```python
from build123d import *

# Parameters (mm, degrees)
SKETCH2_R               = 19.5
BOSS_EXTRUDE1_DEPTH     = 12
SKETCH3_R               = 11
CUT_EXTRUDE1_DEPTH      = 47.5000001
CUT_EXTRUDE1_DEPTH_BACK = 47.5000001
SKETCH4_W               = 8
SKETCH4_H               = 28
CUT_EXTRUDE2_DEPTH      = 47.5000001


with BuildPart() as part:
    # Sketch1 → Revolve1 (revolve)
    with BuildSketch(Plane.XY):
        with BuildLine():
            Line((-46.5, -5.81), (-46.5, -7.81))
            Line((-46.5, -7.81), (-42.5, -7.81))
            Line((-42.5, -7.81), (-42.5, -10.81))
            Line((-42.5, -10.81), (-46.5, -10.81))
            Line((-46.5, -10.81), (-46.5, -12.81))
            Line((-46.5, -12.81), (-42.5, -12.81))
            Line((-42.5, -12.81), (-42.5, -15.81))
            Line((-42.5, -15.81), (-46.5, -15.81))
            Line((-46.5, -15.81), (-46.5, -17.81))
            Line((-46.5, -17.81), (-42.5, -17.81))
            Line((-42.5, -17.81), (-42.5, -20.81))
            Line((-42.5, -20.81), (-46.5, -20.81))
            Line((-46.5, -20.81), (-46.5, -22.81))
            Line((-46.5, -22.81), (-42.5, -22.81))
            Line((-42.5, -22.81), (-42.5, -25.81))
            Line((-42.5, -25.81), (-46.5, -25.81))
            Line((-46.5, -25.81), (-46.5, -63.81))
            Line((-46.5, -63.81), (-42.5, -63.81))
            Line((-42.5, -63.81), (-42.5, -65.81))
            Line((-42.5, -65.81), (-46.5, -65.81))
            Line((-46.5, -65.81), (-46.5, -70.81))
            Line((-46.5, -70.81), (-37, -70.81))
            Line((-37, -70.81), (-37, -8.81))
            Line((-37, -8.81), (0, -8.81))
            Line((0, -8.81), (0, 0))
            ThreePointArc((0, 0), (-23.430767144, -1.458240584), (-46.5, -5.81))
        make_face()
    revolve(axis=Axis((0, 75.597559419, 0), (0, -1, 0)))

    # Sketch2 → Boss-Extrude1 (add)
    with BuildSketch(Plane.XY.offset(25)):
        with Locations((0, -43.81)):
            Circle(SKETCH2_R)
    boss_extrude1 = extrude(amount=BOSS_EXTRUDE1_DEPTH)

    # Mirror1: Boss-Extrude1 across plane
    add(boss_extrude1.mirror(Plane.XY))

    # Sketch3 → Cut-Extrude1 (cut, two sides)
    with BuildSketch(Plane.XY) as cut_extrude1_sk:
        with Locations((0, -43.81)):
            Circle(SKETCH3_R)
    extrude(amount=CUT_EXTRUDE1_DEPTH, mode=Mode.SUBTRACT)
    extrude(cut_extrude1_sk.sketch, amount=-CUT_EXTRUDE1_DEPTH_BACK, mode=Mode.SUBTRACT)

    # Sketch4 → Cut-Extrude2 (cut, symmetric)
    with BuildSketch(Plane(origin=(0, 0, 0), x_dir=(0, 0, -1), z_dir=(1, 0, 0))):
        with Locations((46.5, -43.81)):
            Rectangle(SKETCH4_W, SKETCH4_H)
    cut_extrude2 = extrude(amount=CUT_EXTRUDE2_DEPTH, both=True, mode=Mode.SUBTRACT)

    # Mirror2: Cut-Extrude2 across plane
    add(cut_extrude2.mirror(Plane.XY), mode=Mode.SUBTRACT)


solid = part.part
```
The model under review builds one solid part; all positions refer to its coordinate system, in mm. A direction names the side the tool comes from. Round coordinates to 2 decimals unless told otherwise and drop trailing zeros. Loops run counter-clockwise (first coordinate to the right, second up) from the corner with the lowest first, then second, coordinate; pieces in that order, holes last. Notation, with made-up numbers: M 2.25,7 L 47.25,7 A26 ccw 47.25,23 Z; hole C 73,-13 d7. An arc over 180 degrees is marked long. Answer as a JSON object with one key per item and string values.
(1) Take a section at B-B on y = -43.81. Give the boundary of the cut face in (x, z).
Resolved:
{"outline": "M -19.5,-31.44 A37 cw -19.5,31.44 L -19.5,25 L -11,25 L -11,42.5 L -18.87,42.5 A46.5 ccw -18.87,-42.5 L -11,-42.5 L -11,-25 L -19.5,-25 Z; M 11,-42.5 L 18.87,-42.5 A46.5 ccw 18.87,42.5 L 11,42.5 L 11,25 L 19.5,25 L 19.5,31.44 A37 cw 19.5,-31.44 L 19.5,-25 L 11,-25 Z"}
(2) To check wall thickness, follow line 1 along X through (y, z) = (-55, 0); line 2 along Z through (x, y) = (12.5, -34.5); line 3 along X through (y, z) = (-43, 31). State the ranges of each line that lie inside material, in increasing order.
Resolved:
{"line 1": "-46.5 to -37, 37 to 46.5", "line 2": "-42.5 to -25, 25 to 42.5", "line 3": "-34.66 to -20.2, -19.48 to -10.97, 10.97 to 19.48, 20.2 to 34.66"}
(3) Clearance check with flat-ended pins moving along their axes: P1, Ø11.5, axis at x = -2, y = -36, coming from the +Z side; P2, Ø3, axis at x = 11.5, y = -62, coming from the -Z side; P3, Ø1, axis at y = -36.5, z = 4.5, coming from the +X side. State where each tip first meets the part, or that it passes through.
Resolved:
{"P1": "z = 42.5", "P2": "z = -45.41", "P3": "x = 46.33"}
(4) Take a section at C-C on x = 2. Count the separate pieces of the cut face and the enclosed holes in it, and give its area (3 significant figures).
Resolved:
{"separate pieces": "3", "enclosed holes": "0", "area": "1,650 mm²"}
(5) Tool access review of faces 1 (the flat face through (-20, -12.81, 38)), 2 (the flat face through (0, -29.81, -44)), 3 (the flat face through (8, -52, -25)): name each direction out of +Z, -Z, +X, -X, +Y, -Y from which nothing blocks a thin tool from reaching the whole face with its end or side.
Resolved:
{"face 1": "none", "face 2": "-Z, +X, -X", "face 3": "-Y"}
(6) Take a section at A-A on y = -56.5. Give the boundary of the cut face in (x, z).
Resolved:
{"outline": "M -18.87,-42.5 L 18.87,-42.5 A46.5 ccw 18.87,42.5 L -18.87,42.5 A46.5 ccw Z; hole M -14.81,-33.91 L -14.81,-25 L 14.81,-25 L 14.81,-33.91 A37 ccw 14.81,33.91 L 14.81,25 L -14.81,25 L -14.81,33.91 A37 ccw Z"}
(7) Draft analysis for pull direction Y (two halves, no side actions). For faces 4 (the flat face through (0, -32, -42.5)), 5 (the cylindrical face through (-44.35, -21.82, -13.97)), 6 (the flat face through (0, -57.81, -44)), state which applies: released by +Y, released by -Y, zero draft, split by the parting line, or undercut.
Resolved:
{"face 4": "undercut", "face 5": "zero draft", "face 6": "undercut"}
